```python
from build123d import *

# Parameters (mm, degrees)
SKETCH1_R                 = 19
SKETCH1_R_2               = 11
BOSS_EXTRUDE1_DEPTH       = 3
SKETCH2_R                 = 12
SKETCH2_R_2               = 11
BOSS_EXTRUDE2_DEPTH       = 14
SKETCH3_R                 = 12
SKETCH3_R_2               = 6.5
BOSS_EXTRUDE3_DEPTH       = 1.25
M3_CLEARANCE_HOLE1_D      = 3.2
M3_CLEARANCE_HOLE1_DEPTH  = 7.5
M3_CLEARANCE_HOLE1_TIP    = 0.96137699
M4X0_7_TAPPED_HOLE1_D     = 3.3
M4X0_7_TAPPED_HOLE1_DEPTH = 3


with BuildPart() as part:
    # Sketch1 → Boss-Extrude1 (new body)
    with BuildSketch(Plane(origin=(0, 0, 0), x_dir=(1, 0, 0), z_dir=(0, 1, 0))):
        Circle(SKETCH1_R)
        Circle(SKETCH1_R_2, mode=Mode.SUBTRACT)
    extrude(amount=BOSS_EXTRUDE1_DEPTH)

    # Sketch2 → Boss-Extrude2 (add)
    with BuildSketch(Plane(origin=(0, 3, 0), x_dir=(1, 0, 0), z_dir=(0, 1, 0))):
        Circle(SKETCH2_R)
        Circle(SKETCH2_R_2, mode=Mode.SUBTRACT)
    extrude(amount=BOSS_EXTRUDE2_DEPTH)

    # Sketch3 → Boss-Extrude3 (add)
    with BuildSketch(Plane(origin=(0, 17, 0), x_dir=(1, 0, 0), z_dir=(0, 1, 0))):
        Circle(SKETCH3_R)
        Circle(SKETCH3_R_2, mode=Mode.SUBTRACT)
    extrude(amount=-BOSS_EXTRUDE3_DEPTH)

    # M3 Clearance Hole1
    with Locations(Plane(origin=(0, 17, 0), x_dir=(1, 0, 0), z_dir=(0, 1, 0))):
        with Locations((-7.25, 4.185868355), (7.25, 4.185868355), (0, -8.3715)):
            Hole(M3_CLEARANCE_HOLE1_D / 2, depth=M3_CLEARANCE_HOLE1_DEPTH)
            with Locations((0, 0, -(M3_CLEARANCE_HOLE1_DEPTH + M3_CLEARANCE_HOLE1_TIP / 2))):  # 118° drill point
                Cone(0, M3_CLEARANCE_HOLE1_D / 2, M3_CLEARANCE_HOLE1_TIP, mode=Mode.SUBTRACT)

    # M4x0.7 Tapped Hole1
    with Locations(Plane(origin=(0, 3, 0), x_dir=(1, 0, 0), z_dir=(0, 1, 0))):
        with Locations((-7.75, 13.423393759), (-7.75, -13.423393759), (15.5, 0)):
            Hole(M4X0_7_TAPPED_HOLE1_D / 2, depth=M4X0_7_TAPPED_HOLE1_DEPTH)


solid = part.part
```
Can you work these out from the model? Positions are in its coordinate system, mm. A direction names the side the tool comes from. Give positions to 0.01 mm unless a question says otherwise; leave off trailing zeros. Order: outer loops, then holes, each group sorted by start corner. A loop starts at its lowest first (then second) coordinate and runs counter-clockwise, first axis right, second up. Notation, with made-up numbers: M 21,-26.75 L 72,-26.75 A30 cw 72,12.25 Z; hole C 11.5,56.5 d7. An arc over 180 degrees is marked long. One line per item, written item: value.
1) For P1, Ø4.5, axis at x = -7.75, z = -13.42, coming from the +Y side; P2, Ø3, axis at x = -7.25, z = -4.19, coming from the -Y side; P3, Ø6, axis at x = -7, y = 10.5, coming from the +Z side; P4, Ø10, axis at x = -1, y = 14.5, coming from the +Z side, each with a flat end and sliding along its axis, tell me the tip position at first contact or that it passes through.
Answer sheet:
P1: stops at y = 3
P2: passes through
P3: stops at z = 11.31
P4: stops at z = 12
2) I want a section at D-D, the plane z = 7.5. List the corners of the cut face in (x, y) for me, plus the area to 3 significant figures.
Answer sheet:
outline: M -17.46,0 L -8.05,0 L -8.05,15.75 L -1.34,15.75 L -1.34,17 L -9.37,17 L -9.37,3 L -17.46,3 Z; M 1.34,15.75 L 8.05,15.75 L 8.05,0 L 17.46,0 L 17.46,3 L 9.37,3 L 9.37,17 L 1.34,17 Z
area: 110 mm^2
3) I want a section at B-B, the plane x = 15. List the corners of the cut face in (y, z) for me.
Answer sheet:
outline: M 0,-11.66 L 3,-11.66 L 3,-1.57 L 0,-1.57 Z; M 0,1.57 L 3,1.57 L 3,11.66 L 0,11.66 Z
4) Please list where these lines run through material, in increasing order: line 1 along X through (y, z) = (11, 0); line 2 along Z through (x, y) = (-7.75, 1.8); line 3 along Y through (x, z) = (7.5, -8).
Answer sheet:
line 1: x = -12 to -11, 11 to 12
line 2: z = -17.35 to -15.07, -11.77 to -7.81, 7.81 to 11.77, 15.07 to 17.35
line 3: y = 15.75 to 17
5) I want a section at C-C, the plane x = -7.25. List the corners of the cut face in (y, z) for me.
Answer sheet:
outline: M 0,-17.56 L 3,-17.56 L 3,-15 L 0,-15 Z; M 0,-11.85 L 3,-11.85 L 3,-9.56 L 17,-9.56 L 17,-5.79 L 15.75,-5.79 L 15.75,-8.27 L 0,-8.27 Z; M 0,8.27 L 15.75,8.27 L 15.75,-2.59 L 17,-2.59 L 17,9.56 L 3,9.56 L 3,11.85 L 0,11.85 Z; M 0,15 L 3,15 L 3,17.56 L 0,17.56 Z
6) We'd pull the mould along X, two halves only. Please class faces 1 (the face through (13.976, 1.479, 0.632)), 2 (the face through (-11.99, 9.9, -0.53)), 3 (the face through (12.4, 3, -0.3)): released by +X, released by -X, zero draft, split by the parting line, or undercut.
Answer sheet:
face 1: undercut
face 2: split by the parting line
face 3: zero draft
7) I want a section at A-A, the plane z = 0. List the corners of the cut face in (x, y) for me.
Answer sheet:
outline: M -19,0 L -11,0 L -11,15.75 L -6.5,15.75 L -6.5,17 L -12,17 L -12,3 L -19,3 Z; M 6.5,15.75 L 11,15.75 L 11,0 L 13.85,0 L 13.85,3 L 12,3 L 12,17 L 6.5,17 Z; M 17.15,0 L 19,0 L 19,3 L 17.15,3 Z
8) On a 3-axis mill with a long thin cutter (end or side, diameter ignored), from which of +Z, -Z, +X, -X, +Y, -Y can I reach the whole of each face in a straight line? I mean faces 4 (the face through (-6.1, 16.4, -5.3)), 5 (the face through (-2.38, 7.76, 10.74)). Say none if no direction works.
Answer sheet:
face 4: +Y, -Y
face 5: -Y
